Work out the finished part from the listing and answer in its coordinate system (mm). A direction names the side the tool comes from. Give positions to 0.01 mm unless a question says otherwise; leave off trailing zeros. Write each loop counter-clockwise with the first axis right and the second up, starting at its lowest first coordinate (ties: lowest second). Pieces come first, ordered by that corner, then holes.
1) Given pin 1 Ø8 at (x, z) = (34.5, -46.5) entering from -Y; pin 2 Ø5 at (x, y) = (84.5, -5.5) entering from +Z; pin 3 Ø6 at (x, y) = (86, -2.5) entering from +Z, each flat-ended and moving along its own axis, determine where each tip first touches the part or whether it passes through.
2) Find section B-B (x = 0). Determine the outline of the cut face in (y, z).
3) Straight lines are drawn through the part: probe 1 along Z at (x, y) = (0, -8.95); probe 2 along Z at (x, y) = (0, -2); probe 3 along X at (y, z) = (-9.5, -49.5). For each, find the intervals that lie inside material, in ascending order.
4) Find section C-C (y = -6.5). Determine the outline of the cut face in (x, z).
5) Determine the mould class of faces 1 (the face through (-29.076, -9.014, 48.005)), 2 (the face through (24, 0, 2)) for opening direction X: pulls with the +X half, pulls with the -X half, needs draft (parallel to the pull), parting line crosses it, or undercut.
6) Find section A-A (z = 0). Determine the outline of the cut face in (x, y), plus the area to 3 significant figures.
7) Find section D-D (z = -57.5). Determine the outline of the cut face in (x, y), plus the area to 3 significant figures.
8) A tool of negligible diameter and unlimited length cuts with its end or side. For faces 3 (the face through (55, -8, -18)), 4 (the face through (24, -10, 2)), from which of +Z, -Z, +X, -X, +Y, -Y can it reach the whole face along a straight path? Write none if from no direction.
```python
from build123d import *

# Parameters (mm, degrees)
F0_R     = 115
F0_R_2   = 3.05
F1_DEPTH = 10
F2_R     = 4.95
F3_DEPTH = 2


with BuildPart() as f1:
    # F0 (on Front) → F1 (new body)
    with BuildSketch(Plane.XZ):
        Circle(F0_R)
        Circle(F0_R_2, mode=Mode.SUBTRACT)
    extrude(amount=F1_DEPTH)

    # F2 (on face) → F3 (cut)
    with BuildSketch(Plane.XZ.offset(10)):
        with Locations((0, 57.5)):
            Circle(F2_R)
        with Locations((-33.797652, 46.518477)):
            Circle(F2_R)
        with Locations((-54.68575, 17.768477)):
            Circle(F2_R)
        with Locations((-54.68575, -17.768477)):
            Circle(F2_R)
        with Locations((-33.797652, -46.518477)):
            Circle(F2_R)
        with Locations((0, -57.5)):
            Circle(F2_R)
        with Locations((33.797652, -46.518477)):
            Circle(F2_R)
        with Locations((54.68575, -17.768477)):
            Circle(F2_R)
        with Locations((54.68575, 17.768477)):
            Circle(F2_R)
        with Locations((33.797652, 46.518477)):
            Circle(F2_R)
    extrude(amount=-F3_DEPTH, mode=Mode.SUBTRACT)


solid = f1.part
```
Results:
1. pin 1: stops at y = -8
1. pin 2: stops at z = 80.63
1. pin 3: stops at z = 79.6
2. outline: (-10, -115) - (0, -115) - (0, -3.05) - (-10, -3.05) - (-10, -52.55) - (-8, -52.55) - (-8, -62.45) - (-10, -62.45) - close; (-10, 3.05) - (0, 3.05) - (0, 115) - (-10, 115) - (-10, 62.45) - (-8, 62.45) - (-8, 52.55) - (-10, 52.55) - close
3. probe 1: z = -115 to -62.45, -52.55 to -3.05, 3.05 to 52.55, 62.45 to 115
3. probe 2: z = -115 to -3.05, 3.05 to 115
3. probe 3: x = -103.8 to -37.75, -29.85 to 29.85, 37.75 to 103.8
4. outline: circle Ø230 at (0, 0); hole circle Ø6.1 at (0, 0)
5. face 1: undercut
5. face 2: needs draft
6. outline: (-115, -10) - (-3.05, -10) - (-3.05, 0) - (-115, 0) - close; (3.05, -10) - (115, -10) - (115, 0) - (3.05, 0) - close
6. area: 2,240 mm2
7. outline: (-99.59, -10) - (-4.95, -10) - (-4.95, -8) - (4.95, -8) - (4.95, -10) - (99.59, -10) - (99.59, 0) - (-99.59, 0) - close
7. area: 1,970 mm2
8. face 3: -Y
8. face 4: +Z, -Z, +X, -X, -Y
